The figure shows three views and two pictorial views of one solid part (mm, origin at its lowest corner). Answer the questions. A direction names the side the tool comes from. Round coordinates to 2 decimals unless told otherwise and drop trailing zeros. Order: outer loops, then holes, each group sorted by start corner. A loop starts at its lowest first (then second) coordinate and runs counter-clockwise, first axis right, second up. Notation, with made-up numbers: (14.25, 9) -> (46.25, 9) arc R36 cw to (46.25, 48) -> close; hole circle Ø10 at (-37.75, -8). An arc over 180 degrees is marked (long way). Answer as a JSON object with one key per item and string values. Group by question number.
Item 1: For the marked faces 1 and 2, determine the directions among +Z, -Z, +X, -X, +Y, -Y from which every point of the face is accessible in a straight line to the end or side of a thin tool.
Item 2: Section B-B, the plane x = 4.5 is taken. Write down the section's boundary in (y, z), plus the area to 3 significant figures.
Item 3: Given P1, Ø1, axis at y = 22, z = 4, coming from the -X side; P2, Ø1, axis at x = 8, z = 2, coming from the -Y side, each flat-ended and moving along its own axis, determine where each tip first touches the part or whether it passes through.
Item 4: The mould has two halves that part along Z. Classify the marked faces 3, 4, 5 and 6: pulls with the +Z half, pulls with the -Z half, needs draft (parallel to the pull), parting line crosses it, or undercut.
Item 5: Section D-D, the plane x = 20.5 is taken. Write down the section's boundary in (y, z), plus the area to 3 significant figures.
Item 6: Section C-C, the plane z = 3.75 is taken. Write down the section's boundary in (x, y), plus the area to 3 significant figures.
Item 7: Section A-A, the plane y = 10 is taken. Write down the section's boundary in (x, z).
Item 8: Consider probe 1 along Y at (x, z) = (21.6, 3.75); probe 2 along X at (y, z) = (2.1, 3.75); probe 3 along X at (y, z) = (16.5, 5.5). Determine where each line is inside the solid, lowest interval first. Write a range as from..to.
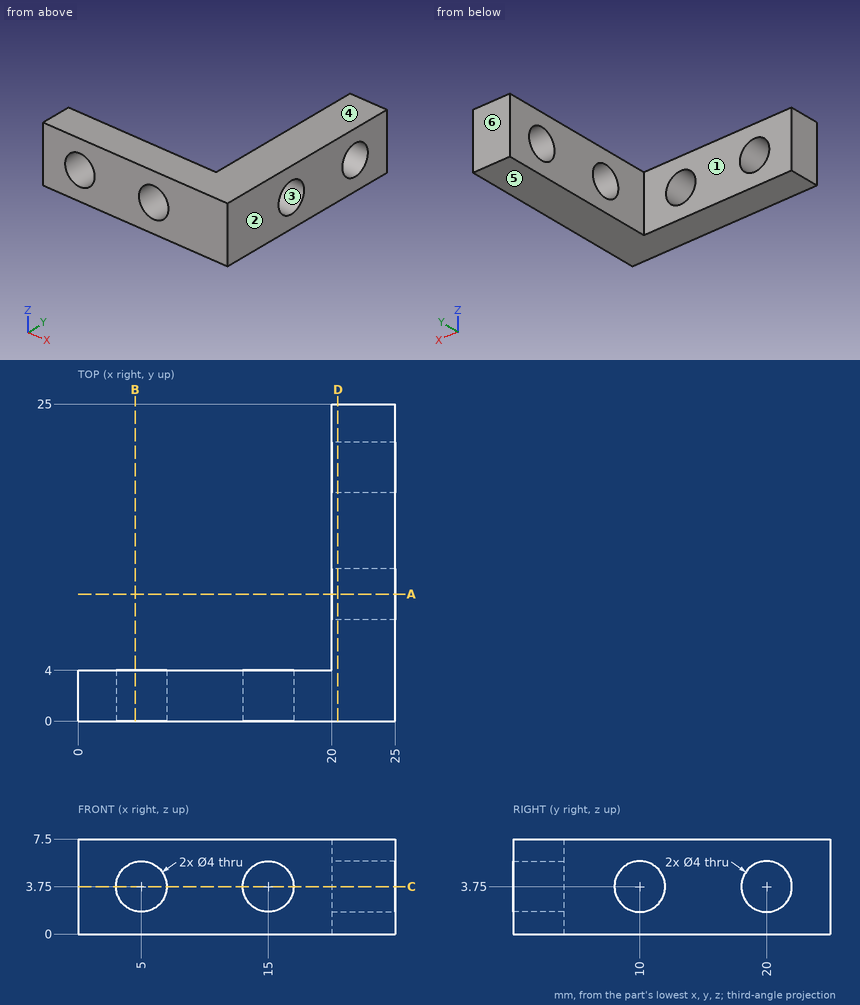
Values found:
{
 "1": {"face 1": "+Z, -Z, -X, +Y", "face 2": "+Z, -Z, +X, +Y, -Y"},
 "2": {"outline": "(0, 0) -> (4, 0) -> (4, 1.81) -> (0, 1.81) -> close; (0, 5.69) -> (4, 5.69) -> (4, 7.5) -> (0, 7.5) -> close", "area": "14.5 mm2"},
 "3": {"P1": "x = 20", "P2": "y = 0"},
 "4": {"face 3": "undercut", "face 4": "pulls with the +Z half", "face 5": "pulls with the -Z half", "face 6": "needs draft"},
 "5": {"outline": "(0, 0) -> (25, 0) -> (25, 7.5) -> (0, 7.5) -> close; hole circle Ø4 at (10, 3.75); hole circle Ø4 at (20, 3.75)", "area": "162 mm2"},
 "6": {"outline": "(0, 0) -> (3, 0) -> (3, 4) -> (0, 4) -> close; (7, 0) -> (13, 0) -> (13, 4) -> (7, 4) -> close; (17, 0) -> (25, 0) -> (25, 8) -> (20, 8) -> (20, 4) -> (17, 4) -> close; (20, 12) -> (25, 12) -> (25, 18) -> (20, 18) -> close; (20, 22) -> (25, 22) -> (25, 25) -> (20, 25) -> close", "area": "133 mm2"},
 "7": {"outline": "(20, 0) -> (25, 0) -> (25, 1.75) -> (20, 1.75) -> close; (20, 5.75) -> (25, 5.75) -> (25, 7.5) -> (20, 7.5) -> close"},
 "8": {"probe 1": "0..8, 12..18, 22..25", "probe 2": "0..3, 7..13, 17..25", "probe 3": "20..25"}
}
